Answer from the drawing. Dimensions are ordinates in mm from the lowest x, y and z of the part. A direction names the side the tool comes from. Coordinates: 2 decimals unless noted, no trailing zeros. Write each loop counter-clockwise with the first axis right and the second up, starting at its lowest first coordinate (ties: lowest second). Pieces come first, ordered by that corner, then holes. Notation, with made-up numbers: (42.5, 40) -> (60.5, 40) arc R17 cw to (60.5, 53) -> close; hole circle Ø3 at (57.25, 62). An arc over 180 degrees is marked (long way). Return JSON: item names as keys, results as strings.
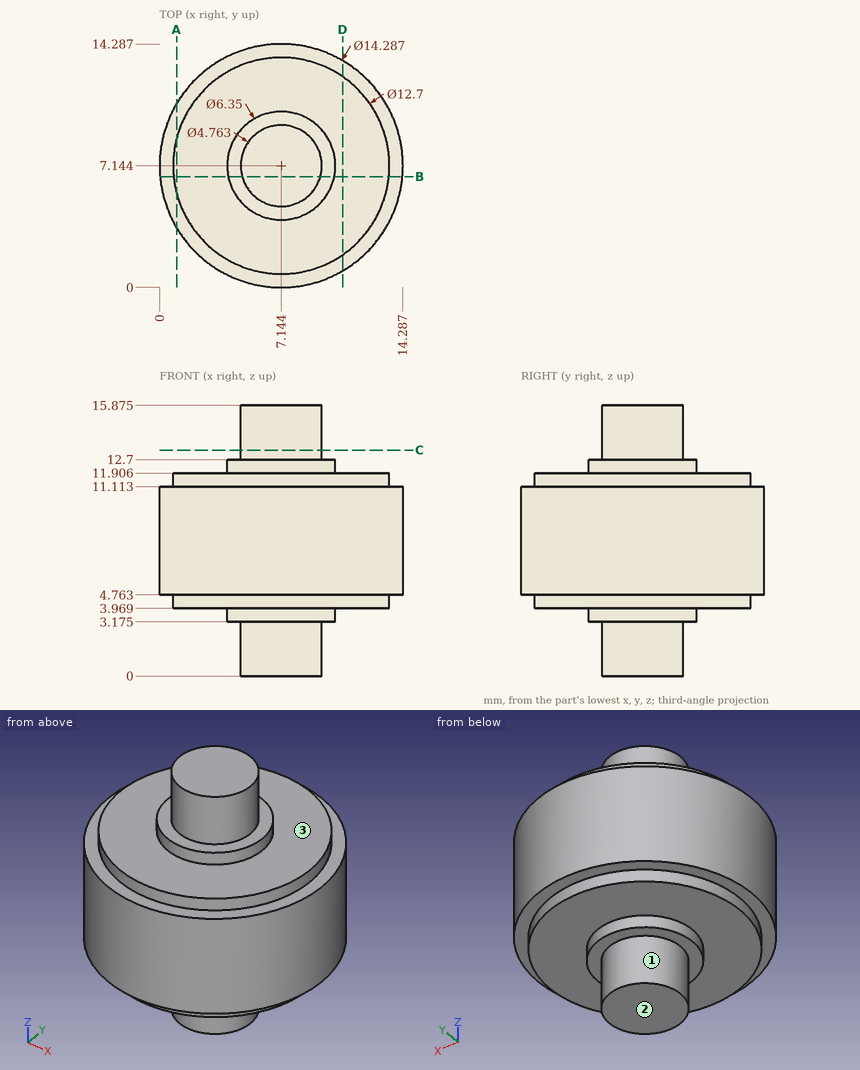
1. A tool of negligible diameter and unlimited length cuts with its end or side. For the marked faces 1, 2 and 3, from which of +Z, -Z, +X, -X, +Y, -Y can it reach the whole face along a straight path? Write none if from no direction.
Taken from the geometry:
{"face 1": "-Z", "face 2": "-Z, +X, -X, +Y, -Y", "face 3": "+Z"}
2. The part is cut by section D-D (x = 10.75). Determine the outline of the cut face in (y, z).
Taken from the geometry:
{"outline": "(0.98, 4.76) -> (1.92, 4.76) -> (1.92, 3.97) -> (12.37, 3.97) -> (12.37, 4.76) -> (13.31, 4.76) -> (13.31, 11.11) -> (12.37, 11.11) -> (12.37, 11.91) -> (1.92, 11.91) -> (1.92, 11.11) -> (0.98, 11.11) -> close"}
3. The part is cut by section C-C (z = 13.25). Determine the outline of the cut face in (x, y) (1 decimal), then the cut area to 3 significant figures.
Taken from the geometry:
{"outline": "circle Ø4.8 at (7.1, 7.1)", "area": "17.8 mm2"}
4. The part is cut by section A-A (x = 1). Determine the outline of the cut face in (y, z), then the cut area to 3 significant figures.
Taken from the geometry:
{"outline": "(3.5, 4.76) -> (5.54, 4.76) -> (5.54, 3.97) -> (8.75, 3.97) -> (8.75, 4.76) -> (10.79, 4.76) -> (10.79, 11.11) -> (8.75, 11.11) -> (8.75, 11.91) -> (5.54, 11.91) -> (5.54, 11.11) -> (3.5, 11.11) -> close", "area": "51.4 mm2"}
5. The part is cut by section B-B (y = 6.5). Determine the outline of the cut face in (x, z) (1 decimal).
Taken from the geometry:
{"outline": "(0, 4.8) -> (0.8, 4.8) -> (0.8, 4) -> (4, 4) -> (4, 3.2) -> (4.9, 3.2) -> (4.9, 0) -> (9.4, 0) -> (9.4, 3.2) -> (10.3, 3.2) -> (10.3, 4) -> (13.5, 4) -> (13.5, 4.8) -> (14.3, 4.8) -> (14.3, 11.1) -> (13.5, 11.1) -> (13.5, 11.9) -> (10.3, 11.9) -> (10.3, 12.7) -> (9.4, 12.7) -> (9.4, 15.9) -> (4.9, 15.9) -> (4.9, 12.7) -> (4, 12.7) -> (4, 11.9) -> (0.8, 11.9) -> (0.8, 11.1) -> (0, 11.1) -> close"}
6. Flat-ended cylindrical pins translate along their axes: pin 1 Ø1.5 at (x, z) = (10, 7.5) entering from +Y; pin 2 Ø1.5 at (x, z) = (12.5, 6.5) entering from +Y (1 decimal); pin 3 Ø1 at (y, z) = (13, 2) entering from -X; pin 4 Ø3 at (y, z) = (9, 9.5) entering from -X. Find the tip coordinate at first contact, or state that the pin passes through.
Taken from the geometry:
{"pin 1": "stops at y = 13.97", "pin 2": "stops at y = 12.6", "pin 3": "passes through", "pin 4": "stops at x = 0.01"}
7. Consider L1, parallel to Y at x = 7, z = 3; L2, parallel to X at y = 7.25, z = 2.25 (1 decimal); L3, parallel to Z at x = 5.25, y = 1. Determine where each line is inside the solid, lowest interval first.
Taken from the geometry:
{"L1": "y = 4.77 to 9.52", "L2": "x = 4.8 to 9.5", "L3": "z = 4.76 to 11.11"}
